Geometry: final body of the model. Coordinates: model frame, mm. A direction names the side the tool comes from. Give positions to 0.01 mm unless a question says otherwise; leave off trailing zeros. Write each loop counter-clockwise with the first axis right and the second up, starting at its lowest first coordinate (ties: lowest second). Pieces come first, ordered by that corner, then holes.
Q1. Pin query (flat end, axial travel): pin 1 Ø4 at (x, y) = (27, 15.5) entering from -Z; pin 2 Ø1.2 at (y, z) = (2, -9.5) entering from +X. Return the tip coordinate at first contact, or that it passes through.
Q2. Mould query, pull axis X, two halves, no side actions, for faces 1 (the flat face through (17, 11, 0)), 2 (the cylindrical face through (1.113, 4.283, -15.826)), 3 (the flat face through (0, 9, -10)). Classes: +X half, -X half, draft (parallel to the pull), parting line (faces both ways), or undercut.
Q3. Line query: line 1 (Y direction, x = 22.1, z = 0.75); line 2 (Y direction, x = 43.55, z = -24); line 3 (X direction, y = 7.5, z = -24.5). Output: solid intervals per line, ascending.
Q4. Section D-D (z = -16.75). Return the cut outline in (x, y), plus the area to 3 significant figures.
Q5. Section C-C (y = 15.75). Return the cut outline in (x, z), plus the area to 3 significant figures.
Q6. Section A-A (z = -4). Return the cut outline in (x, y), plus the area to 3 significant figures.
Q7. Section B-B (x = 29.1). Return the cut outline in (y, z).
Q8. Reachability of faces 4 (the cylindrical face through (1.113, 18.283, -15.826)), 5 (the cylindrical face through (1.014, 18.522, -22.892)), 6 (the cylindrical face through (43.1, 2.6, -8.7)) from +Z, -Z, +X, -X, +Y, -Y: full face, straight path, thin tool, end or side. Return the list, or none.
Autodesk Inventor part; units mm, degrees
ref_plane "YZ Plane" through (0, 0, 0) normal (1, 0, 0) x (0, 1, 0)
ref_plane "XZ Plane" through (0, 0, 0) normal (0, 1, 0) x (-1, 0, 0)
ref_plane "XY Plane" through (0, 0, 0) normal (0, 0, 1) x (1, 0, 0)
sketch "Sketch1" plane through (0, 0, 0) normal (0, 0, 1) x (1, 0, 0)
  line L0 (0, 0) -> (44.2, 0)
  line L1 (44.2, 0) -> (44.2, 21.8)
  line L2 (44.2, 21.8) -> (0, 21.8)
  line L3 (0, 21.8) -> (0, 0)
  dimension "d0" = 21.8
  dimension "d1" = 44.2
extrude "Extrusion1" add sketch "Sketch1" along normal blind 2
sketch "Sketch2" plane through (0, 0, 0) normal (0, 0, -1) x (-1, 0, 0)
  line L0 (0, 21.8) -> (-2, 21.8)
  line L1 (-2, 21.8) -> (-2, 0)
  line L2 (-2, 0) -> (0, 0)
  line L3 (0, 0) -> (0, 21.8)
  line L4 (-44.2, 0) -> (-44.2, 21.8)
  line L5 (0, 0) -> (-44.2, 0)
  line L6 (-44.2, 21.8) -> (-42.2, 21.8)
  line L7 (-42.2, 21.8) -> (-42.2, 0)
  line L8 (-42.2, 0) -> (-44.2, 0)
  line L9 (-44.2, 0) -> (-44.2, 21.8)
  dimension "d4" = 2
  dimension "d5" = 2
  dimension "d93" = 21.8
extrude "Extrusion2" add sketch "Sketch2" along normal blind 26
fillet "Fillet1" radius 10.9 2 edges at (1, 21.8, -26) (1, 0, -26)
fillet "Fillet2" radius 2 2 edges at (43.2, 21.8, -26) (43.2, 0, -26)
sketch "Sketch3" plane through (0, 0, 2) normal (-1, 0, 0) x (0, 0, 1)
  line L0 (-28, 19.8) -> (-28, 2)
  circle A0 centre (-18.75, 10.9) radius 7
  circle A1 centre (-25.75, 10.9) radius 1
  circle A2 centre (-18.75, 3.9) radius 1
  circle A3 centre (-11.75, 10.9) radius 1
  circle A4 centre (-18.75, 17.9) radius 1
  point P0 (-2, 0)
  dimension "d11" = 14
  dimension "d12" = 2
  dimension "d15" = 360
hole "Hole1" at (0, 17.9, -16.75) at (0, 10.9, -23.75) at (0, 3.9, -16.75) at (0, 10.9, -9.75) direction (1, 0, 0) diameter 2 depth 2
thread "Thread1"
thread "Thread2"
thread "Thread3"
thread "Thread4"
sketch "Sketch4" plane through (44.2, 0, 2) normal (1, 0, 0) x (0, 0, -1)
  line L0 (26, 21.8) -> (0, 21.8)
  arc A0 (28, 19.8) -> (26, 21.8) centre (26, 19.8) ccw
  circle A1 centre (11.5, 19.8) radius 1
  circle A2 centre (26, 19.8) radius 1
  line L1 (26, 0) -> (26, 2)
  circle A3 centre (26, 2) radius 1
  circle A4 centre (11.5, 2) radius 1
  point P0 (2, 0)
  dimension "d34" = 2
  dimension "d35" = 2
  dimension "d36" = 2
  dimension "d37" = 2
  dimension "d38" = 2
hole "Hole2" at (44.2, 19.8, -9.5) at (44.2, 19.8, -24) at (44.2, 2, -24) at (44.2, 2, -9.5) direction (-1, 0, 0) diameter 2 depth 2
thread "Thread5"
thread "Thread6"
thread "Thread7"
thread "Thread8"
fillet "Fillet3" radius 2 2 edges at (0, 10.9, 2) (44.2, 10.9, 2)
sketch "Sketch5" plane through (0, 21.8, -15.1) normal (-1, 0, 0) x (0, 0, 1)
  circle A0 centre (-1.65, -3.9) radius 1
  circle A1 centre (-1.65, -17.9) radius 1
  line L0 (-1.65, -3.9) -> (-1.65, -17.9)
  circle A2 centre (-1.65, -10.9) radius 4
  point P0 (15.1, -21.8)
  dimension "d55" = 8
hole "Hole3" at (0, 10.9, -16.75) direction (1, 0, 0) diameter 8 depth 44.75
sketch "Sketch6" plane through (0, 0, 2) normal (0, 0, 1) x (1, 0, 0)
  line L0 (2, 0) -> (42.2, 0)
  line L1 (22.1, 0) -> (22.1, 21.8)
  line L2 (42.2, 21.8) -> (2, 21.8)
  line L3 (44.4097, 10.9) -> (-11.7207, 10.9)
  circle A0 centre (22.1, 10.9) radius 3
  circle A1 centre (22.1, 10.9) radius 7
  circle A2 centre (22.1, 3.9) radius 1
  circle A3 centre (29.1, 10.9) radius 1
  circle A4 centre (22.1, 17.9) radius 1
  circle A5 centre (15.1, 10.9) radius 1
  point P0 (0, 0)
  dimension "d64" = 14
  dimension "d63" = 6
  dimension "d65" = 2
  dimension "d68" = 360
hole "Hole4" at (22.1, 3.9, 2) at (29.1, 10.9, 2) at (22.1, 17.9, 2) at (15.1, 10.9, 2) direction (0, 0, -1) diameter 2 depth 2
sketch "Sketch7" plane through (0, 0, 2) normal (0, 0, 1) x (1, 0, 0)
  circle A0 centre (22.1, 3.9) radius 1
  circle A1 centre (22.1, 17.9) radius 1
  line L0 (22.1, 3.9) -> (22.1, 17.9)
  circle A2 centre (22.1, 10.9) radius 3
  point P0 (0, 0)
  dimension "d77" = 6
hole "Hole5" at (22.1, 10.9, 2) direction (0, 0, -1) diameter 6 depth 2
thread "Thread9"
thread "Thread10"
thread "Thread11"
thread "Thread12"
chamfer "Chamfer1" distance 0.2 angle 45 12 edges at (44.2, 2, -8.5) (44.2, 19.8, -8.5) (44.2, 2, -23) (44.2, 19.8, -23) (22.1, 4.9, 2) (15.1, 11.9, 2) (29.1, 11.9, 2) (22.1, 18.9, 2) (0, 10.9, -10.75) (0, 17.9, -17.75) (0, 3.9, -17.75) (0, 10.9, -24.75)
Computed:
1. pin 1: stops at z = 0
1. pin 2: stops at x = 2
2. face 1: undercut
2. face 2: draft
2. face 3: -X half
3. line 1: y = 0 to 2.9, 4.9 to 7.9, 13.9 to 16.9, 18.9 to 21.8
3. line 2: y = 0 to 1, 3 to 18.8, 20.8 to 21.8
3. line 3: x = 0 to 2, 42.2 to 44.2
4. outline: (0, 0.13) - (2, 0.13) - (2, 2.9) - (0.2, 2.9) - (0, 2.7) - close; (0, 5.1) - (0.2, 4.9) - (2, 4.9) - (2, 6.9) - (0, 6.9) - close; (0, 14.9) - (2, 14.9) - (2, 16.9) - (0.2, 16.9) - (0, 16.7) - close; (0, 19.1) - (0.2, 18.9) - (2, 18.9) - (2, 21.67) - (0, 21.67) - close; (42.2, 0) - (44.2, 0) - (44.2, 6.9) - (42.2, 6.9) - close; (42.2, 14.9) - (44.2, 14.9) - (44.2, 21.8) - (42.2, 21.8) - close
4. area: 46.6 mm2
5. outline: (0, -24.86) - (2, -24.86) - (2, 0) - (42.2, 0) - (42.2, -26) - (44.2, -26) - (44.2, 0) arc R2 ccw to (42.2, 2) - (2, 2) arc R2 ccw to (0, 0) - close
5. area: 188 mm2
6. outline: (0, 0) - (2, 0) - (2, 21.8) - (0, 21.8) - close; (42.2, 0) - (44.2, 0) - (44.2, 21.8) - (42.2, 21.8) - close
6. area: 87.2 mm2
7. outline: (0, 0) - (9.9, 0) - (9.9, 1.8) - (9.7, 2) - (0, 2) - close; (11.9, 0) - (21.8, 0) - (21.8, 2) - (12.1, 2) - (11.9, 1.8) - close
8. face 4: -X
8. face 5: -Z, -X, +Y
8. face 6: +X
